from build123d import *

# Parameters (mm, degrees)
F1_DEPTH = 4
F0_W     = 2
F0_H     = 30
F2_DEPTH = 2
F0_W_2   = 4
F3_DEPTH = 3


with BuildPart() as f1:
    # F0 (on Top) → F1 (new body)
    with BuildSketch(Plane.XY):
        Polygon((-6, 5), (-10, 5), (-10, 0), (10, 0), (10, 5), (6, 5), (4, 5), (-4, 5), align=None)
    extrude(amount=F1_DEPTH)

    # F0 (on Top) → F2 (join)
    with BuildSketch(Plane.XY):
        with Locations((-5, 20)):
            Rectangle(F0_W, F0_H)
        with Locations((5, 20)):
            Rectangle(F0_W, F0_H)
    extrude(amount=F2_DEPTH)

    # F0 (on Top) → F3 (join)
    with BuildSketch(Plane.XY):
        with Locations((8, 20)):
            Rectangle(F0_W_2, F0_H)
        with Locations((-8, 20)):
            Rectangle(F0_W_2, F0_H)
    extrude(amount=F3_DEPTH)


solid = f1.part
Geometry: final body of the model. Coordinates: model frame, mm. A direction names the side the tool comes from. Coordinates: 2 decimals unless noted, no trailing zeros. Write each loop counter-clockwise with the first axis right and the second up, starting at its lowest first coordinate (ties: lowest second). Pieces come first, ordered by that corner, then holes. Notation, with made-up numbers: (1, 4) - (53, 4) arc R8 ccw to (53, 18) - close; hole circle Ø5 at (-39.75, 68). An arc over 180 degrees is marked (long way). Return JSON: item names as keys, results as strings.
Item 1: Section query D-D (x = 5). Output: boundary loops of the cut face in (y, z), and give its area (3 significant figures).
Completed:
{"outline": "(0, 0) - (35, 0) - (35, 2) - (5, 2) - (5, 4) - (0, 4) - close", "area": "80.0 mm2"}
Item 2: Reachability of faces 1 (the face through (-7, 35, 1)), 2 (the face through (8, 20, 3)), 3 (the face through (4, 20, 1)), 4 (the face through (5, 20, 2)) from +Z, -Z, +X, -X, +Y, -Y: full face, straight path, thin tool, end or side. Return the list, or none.
Completed:
{"face 1": "+Z, -Z, +X, -X, +Y", "face 2": "+Z, +X, -X, +Y", "face 3": "+Z, -Z, +Y", "face 4": "+Z, +Y"}
Item 3: Section query B-B (z = 1.1). Output: boundary loops of the cut face in (x, y), and give its area (3 significant figures).
Completed:
{"outline": "(-10, 0) - (10, 0) - (10, 35) - (4, 35) - (4, 5) - (-4, 5) - (-4, 35) - (-10, 35) - close", "area": "460 mm2"}
Item 4: Line query: L1, parallel to X at y = 14, z = 1.1; L2, parallel to X at y = 27, z = 2.15; L3, parallel to Z at x = 5, y = 6. Output: solid intervals per line, ascending.
Completed:
{"L1": "x = -10 to -4, 4 to 10", "L2": "x = -10 to -6, 6 to 10", "L3": "z = 0 to 2"}
Item 5: Section query C-C (x = 7.5). Output: boundary loops of the cut face in (y, z).
Completed:
{"outline": "(0, 0) - (35, 0) - (35, 3) - (5, 3) - (5, 4) - (0, 4) - close"}
Item 6: Section query A-A (y = 28). Output: boundary loops of the cut face in (x, z).
Completed:
{"outline": "(-10, 0) - (-4, 0) - (-4, 2) - (-6, 2) - (-6, 3) - (-10, 3) - close; (4, 0) - (10, 0) - (10, 3) - (6, 3) - (6, 2) - (4, 2) - close"}
Item 7: Pin query (flat end, axial travel): pin 1 Ø2 at (x, y) = (8, 24.5) entering from +Z; pin 2 Ø0.6 at (x, y) = (-4.5, 26) entering from +Z. Return the tip coordinate at first contact, or that it passes through.
Completed:
{"pin 1": "stops at z = 3", "pin 2": "stops at z = 2"}
Item 8: Pull-direction query (X, two-part tool) for faces 5 (the face through (7, 35, 1)), 6 (the face through (0, 5, 2)), 7 (the face through (-10, 18, 2)); classes: +X half, -X half, draft (parallel to the pull), parting line (faces both ways), or undercut.
Completed:
{"face 5": "draft", "face 6": "undercut", "face 7": "-X half"}
